Part model, mm, in its own coordinate system. A direction names the side the tool comes from. Give positions to 0.01 mm unless a question says otherwise; leave off trailing zeros. Write each loop counter-clockwise with the first axis right and the second up, starting at its lowest first coordinate (ties: lowest second). Pieces come first, ordered by that corner, then holes.
```python
from build123d import *

# Parameters (mm, degrees)
BOSS_EXTRUDE1_DEPTH  = 3
SKETCH2_R            = 1.5
CUT_EXTRUDE1_DEPTH   = 3
SKETCH3_R            = 30
SKETCH3_R_2          = 15
CUT_EXTRUDE2_DEPTH   = 3
SKETCH4_R            = 18
BOSS_EXTRUDE6_DEPTH  = 3
SKETCH5_R            = 15
BOSS_EXTRUDE7_DEPTH  = 3
SKETCH6_R            = 15.225419419
BOSS_EXTRUDE8_DEPTH  = 3
SKETCH7_R            = 1.5
CUT_EXTRUDE4_DEPTH   = 3
SKETCH9_R            = 10
CUT_EXTRUDE5_DEPTH   = 3
SKETCH10_R           = 19.155501788
BOSS_EXTRUDE9_DEPTH  = 3
SKETCH11_R           = 13.756788871
BOSS_EXTRUDE10_DEPTH = 3
SKETCH12_R           = 11.549228796
BOSS_EXTRUDE11_DEPTH = 3
SKETCH14_R           = 9.610550559
BOSS_EXTRUDE12_DEPTH = 3
SKETCH15_R           = 14.086691916
BOSS_EXTRUDE13_DEPTH = 3
SKETCH16_R           = 15.543730799
BOSS_EXTRUDE14_DEPTH = 3
SKETCH17_R           = 14.681473261
BOSS_EXTRUDE17_DEPTH = 3
SKETCH18_R           = 13.614072274
BOSS_EXTRUDE18_DEPTH = 3
SKETCH19_R           = 1.5
CUT_EXTRUDE6_DEPTH   = 10
SKETCH20_R           = 5
CUT_EXTRUDE8_DEPTH   = 2
CUT_EXTRUDE11_DEPTH  = 14


with BuildPart() as part:
    # Sketch1 → Boss-Extrude1 (new body)
    with BuildSketch(Plane.XY):
        with BuildLine():
            Line((-32.133468612, 81.630943295), (32.133468612, 81.630943295))
            Line((32.133468612, 81.630943295), (81.630943295, 32.133468612))
            Line((81.630943295, 32.133468612), (81.630943295, -32.133468612))
            Line((81.630943295, -32.133468612), (32.133468612, -81.630943295))
            add(Edge.make_bspline(
                [(-32.133468612, -81.630943295), (-26.315604905, -78.929469601), (-17.458466972, -75.90692924), (-6.459846686, -74.366971031), (0.503945588, -74.095540146), (13.381410653, -74.737409183), (24.194527132, -77.919288079), (32.133468612, -81.630943295)],
                knots=[0, 0, 0, 0, 0.289771888, 0.418866631, 0.500125988, 0.604148798, 1, 1, 1, 1], degree=3))
            Line((-32.133468612, -81.630943295), (-81.630943295, -32.133468612))
            Line((-81.630943295, -32.133468612), (-81.630943295, 32.133468612))
            Line((-81.630943295, 32.133468612), (-32.133468612, 81.630943295))
        make_face()
    extrude(amount=BOSS_EXTRUDE1_DEPTH)

    # Sketch2 → Cut-Extrude1 (cut)
    with BuildSketch(Plane.XY.offset(3)):
        with Locations((-39.204536424, -39.204536424)):
            Circle(SKETCH2_R)
        with Locations((39.204536424, -39.204536424)):
            Circle(SKETCH2_R)
        with Locations((39.204536424, 39.204536424)):
            Circle(SKETCH2_R)
        with Locations((-39.204536424, 39.204536424)):
            Circle(SKETCH2_R)
    extrude(amount=-CUT_EXTRUDE1_DEPTH, mode=Mode.SUBTRACT)

    # Sketch3 → Cut-Extrude2 (cut)
    with BuildSketch(Plane.XY.offset(3)):
        Circle(SKETCH3_R)
        with Locations((0, 30)):
            Circle(SKETCH3_R_2)
        Circle(SKETCH3_R)
        with Locations((0, 30)):
            Circle(SKETCH3_R_2)
        with Locations((0, -30)):
            Circle(SKETCH3_R_2)
        Circle(SKETCH3_R)
        with Locations((30, 0)):
            Circle(SKETCH3_R_2)
        with Locations((0, 30)):
            Circle(SKETCH3_R_2)
        with Locations((-30, 0)):
            Circle(SKETCH3_R_2)
        Circle(SKETCH3_R)
        with Locations((-30, 0)):
            Circle(SKETCH3_R_2)
        Circle(SKETCH3_R)
        with Locations((0, -30)):
            Circle(SKETCH3_R_2)
        Circle(SKETCH3_R)
        with Locations((30, 0)):
            Circle(SKETCH3_R_2)
        Circle(SKETCH3_R)
        with Locations((30, 0)):
            Circle(SKETCH3_R_2)
        Circle(SKETCH3_R)
        with Locations((0, -30)):
            Circle(SKETCH3_R_2)
        Circle(SKETCH3_R)
        with Locations((-30, 0)):
            Circle(SKETCH3_R_2)
    extrude(amount=-CUT_EXTRUDE2_DEPTH, mode=Mode.SUBTRACT)

    # Sketch4 → Boss-Extrude6 (add)
    with BuildSketch(Plane.XY.offset(3)):
        with Locations((-35.186247216, 0)):
            Circle(SKETCH4_R)
        with Locations((35.19, 0)):
            Circle(SKETCH4_R)
    extrude(amount=-BOSS_EXTRUDE6_DEPTH)

    # Sketch5 → Boss-Extrude7 (add)
    with BuildSketch(Plane.XY.offset(3)):
        with Locations((0, -30)):
            Circle(SKETCH5_R)
    extrude(amount=-BOSS_EXTRUDE7_DEPTH)

    # Sketch6 → Boss-Extrude8 (add)
    with BuildSketch(Plane.XY.offset(3)):
        with Locations((0, 30)):
            Circle(SKETCH6_R)
    extrude(amount=-BOSS_EXTRUDE8_DEPTH)

    # Sketch7 → Cut-Extrude4 (cut)
    with BuildSketch(Plane.XY.offset(3)):
        with Locations((-46.253324199, 32.134700114)):
            Circle(SKETCH7_R)
        with Locations((-52.103605786, -20.865299886)):
            Circle(SKETCH7_R)
        with Locations((34.896394214, -20.865299886)):
            Circle(SKETCH7_R)
        with Locations((34.896394214, 32.134700114)):
            Circle(SKETCH7_R)
    extrude(amount=-CUT_EXTRUDE4_DEPTH, mode=Mode.SUBTRACT)

    # Sketch9 → Cut-Extrude5 (cut)
    with BuildSketch(Plane.XY.offset(3)):
        with Locations((0, 65.004511024)):
            Circle(SKETCH9_R)
        with Locations((0, -51.773637368)):
            Circle(SKETCH9_R)
        with Locations((-62.186247216, 0)):
            Circle(SKETCH9_R)
        with Locations((62.19, 0)):
            Circle(SKETCH9_R)
    extrude(amount=-CUT_EXTRUDE5_DEPTH, mode=Mode.SUBTRACT)

    # Sketch10 → Boss-Extrude9 (add)
    with BuildSketch(Plane.XY.offset(3)):
        with Locations((-48.672279754, -29.553895966)):
            Circle(SKETCH10_R)
    extrude(amount=-BOSS_EXTRUDE9_DEPTH)

    # Sketch11 → Boss-Extrude10 (add)
    with BuildSketch(Plane.XY.offset(3)):
        with Locations((37.212476286, -30.975829013)):
            Circle(SKETCH11_R)
    extrude(amount=-BOSS_EXTRUDE10_DEPTH)

    # Sketch12 → Boss-Extrude11 (add)
    with BuildSketch(Plane.XY.offset(3)):
        with Locations((38.591163572, 36.494236376)):
            Circle(SKETCH12_R)
    extrude(amount=-BOSS_EXTRUDE11_DEPTH)

    # Sketch14 → Boss-Extrude12 (add)
    with BuildSketch(Plane.XY.offset(3)):
        with Locations((-42.212724403, 37.609741157)):
            Circle(SKETCH14_R)
    extrude(amount=-BOSS_EXTRUDE12_DEPTH)

    # Sketch15 → Boss-Extrude13 (add)
    with BuildSketch(Plane.XY.offset(3)):
        with Locations((0, -51.773637368)):
            Circle(SKETCH15_R)
    extrude(amount=-BOSS_EXTRUDE13_DEPTH)

    # Sketch16 → Boss-Extrude14 (add)
    with BuildSketch(Plane.XY.offset(3)):
        with Locations((-63.76815814, 0)):
            Circle(SKETCH16_R)
    extrude(amount=-BOSS_EXTRUDE14_DEPTH)

    # Sketch17 → Boss-Extrude17 (add)
    with BuildSketch(Plane.XY.offset(3)):
        with Locations((-0.058768436, 63.845084824)):
            Circle(SKETCH17_R)
    extrude(amount=-BOSS_EXTRUDE17_DEPTH)

    # Sketch18 → Boss-Extrude18 (add)
    with BuildSketch(Plane(origin=(0, 0, 0), x_dir=(-1, 0, 0), z_dir=(0, 0, -1))):
        with Locations((-63.543622385, 0)):
            Circle(SKETCH18_R)
    extrude(amount=-BOSS_EXTRUDE18_DEPTH)

    # Sketch19 → Cut-Extrude6 (cut)
    with BuildSketch(Plane(origin=(0, 0, 0), x_dir=(-1, 0, 0), z_dir=(0, 0, -1))):
        with Locations((0, 55)):
            Circle(SKETCH19_R)
        with Locations((55, 0)):
            Circle(SKETCH19_R)
        with Locations((0, -55)):
            Circle(SKETCH19_R)
        with Locations((-55, 0)):
            Circle(SKETCH19_R)
    extrude(amount=-CUT_EXTRUDE6_DEPTH, mode=Mode.SUBTRACT)

    # Sketch20 → Cut-Extrude8 (cut)
    with BuildSketch(Plane(origin=(0, 0, 0), x_dir=(-1, 0, 0), z_dir=(0, 0, -1))):
        with Locations((0, 55)):
            Circle(SKETCH20_R)
        with Locations((55, 0)):
            Circle(SKETCH20_R)
        with Locations((0, -55)):
            Circle(SKETCH20_R)
        with Locations((-55, 0)):
            Circle(SKETCH20_R)
    extrude(amount=-CUT_EXTRUDE8_DEPTH, mode=Mode.SUBTRACT)

    # Sketch21 → Cut-Extrude11 (cut)
    with BuildSketch(Plane(origin=(0, 0, 0), x_dir=(-1, 0, 0), z_dir=(0, 0, -1))):
        with BuildLine():
            add(Edge.make_bspline(
                [(-25.779143223, 15.343916538), (-25.444782602, 17.404426932), (-20.814862678, 21.253079788), (-11.928002545, 31.54538853), (1.317e-05, 2.953987482), (11.927707302, 31.545045431), (20.814157023, 21.253821997), (30.670361401, 13.0612405), (7.851072174, 0.001919986), (30.702175927, -13.101903603), (20.72807921, -21.32903317), (11.794640134, -31.622543771), (1.2848e-05, -3.377971787), (-11.794933778, -31.622888023), (-20.72878866, -21.328293053), (-30.702340419, -13.101151105), (-7.858122441, 0.001919089), (-26.533922641, 10.69255887), (-25.779143223, 15.343916538)],
                knots=[0, 0, 0, 0, 0.037620183, 0.075240365, 0.165070914, 0.254901463, 0.292516948, 0.330132434, 0.415069121, 0.500005809, 0.538178927, 0.576352045, 0.665075111, 0.753798177, 0.791975991, 0.830153805, 0.915076903, 1, 1, 1, 1], degree=3))
        make_face()
    extrude(amount=-CUT_EXTRUDE11_DEPTH, mode=Mode.SUBTRACT)


solid = part.part
```
1) Saw through at A-A, the plane z = 1.35. Count the separate pieces of the cut face and the enclosed holes in it, then the cut area to 3 significant figures.
Answers follow:
separate pieces: 1
enclosed holes: 5
area: 19,200 mm2
2) 3-axis set-ups, long thin cutter, end or side, ignore diameter. For faces 4 (the face through (-57.229, 56.536, 1.479)), 5 (the face through (-53.8, 1.2, 2)): which of +Z, -Z, +X, -X, +Y, -Y reach the whole face in a straight line?
Answers follow:
face 4: +Z, -Z, -X, +Y
face 5: -Z
3) Pin check, flat tips, straight feed: pin 1 Ø6 at (x, y) = (-55, 0) entering from +Z; pin 2 Ø6 at (x, y) = (0, -55) entering from -Z. Stop position of each tip, or through.
Answers follow:
pin 1: stops at z = 3
pin 2: stops at z = 2
4) Wall check: L1, parallel to Y at x = 0, z = 2.5; L2, parallel to Y at x = 0, z = 0.45; L3, parallel to X at y = 3.5, z = 0.7. Give the ranges that are in metal, low to high.
Answers follow:
L1: y = -74.19 to -56.5, -53.5 to -15, 14.77 to 53.5, 56.5 to 81.63
L2: y = -74.19 to -60, -50 to -15, 14.77 to 50, 60 to 81.63
L3: x = -81.63 to -58.57, -51.43 to -18.33, 18.33 to 51.43, 58.57 to 81.63
5) Saw through at B-B, the plane x = -71.5. Write the cut outline in (y, z).
Answers follow:
outline: (-42.26, 0) - (42.26, 0) - (42.26, 3) - (-42.26, 3) - close
6) Two-plate mould, pull along Y, no slides. Class faces 1 (the face through (56.2, 1.2, 2)), 2 (the face through (-56.536, -57.229, 1.479)), 3 (the face through (-1, -17, 3)): +Y half, -Y half, draft (parallel to the pull), parting line (faces both ways), or undercut.
Answers follow:
face 1: undercut
face 2: -Y half
face 3: draft
